Model file for the job. Use its own axes, mm. Face numbers are marked on the shaded views. A direction names the side the tool comes from. Round coordinates to 2 decimals unless told otherwise and drop trailing zeros. Order: outer loops, then holes, each group sorted by start corner. A loop starts at its lowest first (then second) coordinate and runs counter-clockwise, first axis right, second up. Notation, with made-up numbers: (-20.5, -27.5) -> (21.5, -27.5) arc R27 ccw to (21.5, -7.5) -> close; hole circle Ø3 at (57, 26.25). An arc over 180 degrees is marked (long way). Put each result on its own line as item: value. Start each with the question number.
Q1. Cut at B-B, the plane z = 6. List the corners of the cut face in (x, y).
Q2. Cut at D-D, the plane y = 1.5. List the corners of the cut face in (x, z), and give its area (3 significant figures).
Q3. Flat gauge pin, fed straight in: P1, Ø1.5, axis at x = -1, y = -0.5, coming from the +Z side. Where does the tip first touch, or does it go through?
Q4. Probe L1, parallel to X at y = -14.55, z = 6; L2, parallel to Z at x = 0, y = -13.85; L3, parallel to Y at x = 0.9, z = 8.5. List the from-to ranges inside material, lowest first.
Q5. Cut at C-C, the plane z = 8.75. List the corners of the cut face in (x, y).
Q6. 3-axis set-ups, long thin cutter, end or side, ignore diameter. For the marked faces 1 and 2: which of +Z, -Z, +X, -X, +Y, -Y reach the whole face in a straight line?
Q7. Pull direction Y, two halves, no side cores. Call the marked faces 3, 4, 5 and 6: released by +Y, released by -Y, zero draft, split by the parting line, or undercut.
Q8. Cut at A-A, the plane x = 0. List the corners of the cut face in (y, z).
Autodesk Inventor part; units mm, degrees
ref_plane "YZ Plane" through (0, 0, 0) normal (1, 0, 0) x (0, 1, 0)
ref_plane "XZ Plane" through (0, 0, 0) normal (0, 1, 0) x (-1, 0, 0)
ref_plane "XY Plane" through (0, 0, 0) normal (0, 0, 1) x (1, 0, 0)
sketch "Sketch1" plane through (0, 0, 0) normal (0, 0, 1) x (1, 0, 0)
  line L0 (-2.5, 15.2) -> (2.5, 15.2)
  line L1 (2.5, 15.2) -> (2.5, -15.2)
  line L2 (2.5, -15.2) -> (-2.5, -15.2)
  line L3 (-2.5, -15.2) -> (-2.5, 15.2)
  point P0 (0, 0)
  point P1 (2.5, 0)
  point P2 (0, 15.2)
  dimension "d0" = 30.4
  dimension "d1" = 5
extrude "Extrusion1" add sketch "Sketch1" along normal blind 2
sketch "Sketch2" plane through (-2.5, 15.2, 0) normal (0, 1, 0) x (1, 0, 0)
  line L0 (5, -2) -> (0, -2)
  line L1 (0, -2) -> (5, -2)
  line L2 (5, -2) -> (5, -10)
  line L3 (5, -10) -> (0, -10)
  line L4 (0, -10) -> (0, -2)
  point P0 (2.5, 0)
  dimension "d4" = 5
  dimension "d5" = 8
extrude "Extrusion2" add sketch "Sketch2" against normal blind 2
mirror "Mirror1" about plane through (0, 0, 0) normal (0, 1, 0) of "Extrusion2"
sketch "Sketch3" plane through (-2.5, 15.2, 0) normal (0, 1, 0) x (1, 0, 0)
  line L0 (5, -10) -> (0, -10)
  line L1 (5, -2) -> (5, -10)
  line L2 (0, -2) -> (5, -2)
  line L3 (0, -10) -> (0, -2)
  point P0 (2.5, 0)
  point P1 (2.5, -6)
  point P2 (2.5, -2)
  point P3 (0, -6)
hole "Hole1" at (0, 15.2, 6) direction (0, -1, 0) diameter 3.2 depth 30.4
fillet "Fillet1" radius 0.5 8 edges at (0, 15.2, 0) (0, -15.2, 0) (0, -15.2, 10) (0, -13.2, 10) (0, -13.2, 2) (0, 13.2, 2) (0, 13.2, 10) (0, 15.2, 10)
properties part number "bobastacksupport" material "Aluminum 6061"
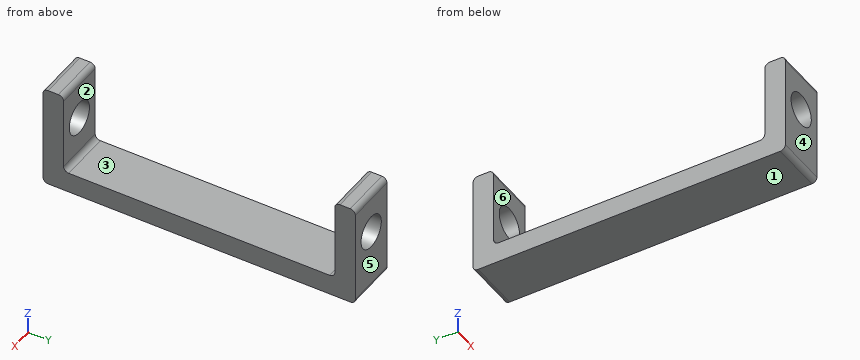
Ans:
1. outline: (-2.5, -15.2) -> (-1.6, -15.2) -> (-1.6, -13.2) -> (-2.5, -13.2) -> close; (-2.5, 13.2) -> (-1.6, 13.2) -> (-1.6, 15.2) -> (-2.5, 15.2) -> close; (1.6, -15.2) -> (2.5, -15.2) -> (2.5, -13.2) -> (1.6, -13.2) -> close; (1.6, 13.2) -> (2.5, 13.2) -> (2.5, 15.2) -> (1.6, 15.2) -> close
2. outline: (-2.5, 0) -> (2.5, 0) -> (2.5, 2) -> (-2.5, 2) -> close
2. area: 10.0 mm^2
3. P1: stops at z = 2
4. L1: x = -2.5 to -1.6, 1.6 to 2.5
4. L2: z = 0 to 4.4, 7.6 to 10
4. L3: y = -15.2 to -13.2, 13.2 to 15.2
5. outline: (-2.5, -15.2) -> (2.5, -15.2) -> (2.5, -13.2) -> (-2.5, -13.2) -> close; (-2.5, 13.2) -> (2.5, 13.2) -> (2.5, 15.2) -> (-2.5, 15.2) -> close
6. face 1: -Z, +X, -X, +Y, -Y
6. face 2: +Z, +X, -X
7. face 3: undercut
7. face 4: released by -Y
7. face 5: released by +Y
7. face 6: undercut
8. outline: (-15.2, 0.5) arc R0.5 ccw to (-14.7, 0) -> (14.7, 0) arc R0.5 ccw to (15.2, 0.5) -> (15.2, 4.4) -> (13.2, 4.4) -> (13.2, 2.5) arc R0.5 cw to (12.7, 2) -> (-12.7, 2) arc R0.5 cw to (-13.2, 2.5) -> (-13.2, 4.4) -> (-15.2, 4.4) -> close; (-15.2, 7.6) -> (-13.2, 7.6) -> (-13.2, 9.5) arc R0.5 ccw to (-13.7, 10) -> (-14.7, 10) arc R0.5 ccw to (-15.2, 9.5) -> close; (13.2, 7.6) -> (15.2, 7.6) -> (15.2, 9.5) arc R0.5 ccw to (14.7, 10) -> (13.7, 10) arc R0.5 ccw to (13.2, 9.5) -> close
